```python
from build123d import *

# Parameters (mm, degrees)
EXTRUDE_1_DEPTH = 3
SKETCH_2_R      = 6.5
EXTRUDE_2_DEPTH = 0.2
SKETCH_4_W      = 3
SKETCH_4_H      = 5
EXTRUDE_3_DEPTH = 1


with BuildPart() as part:
    # 草图1 → 凸台-拉伸1 (new body)
    with BuildSketch(Plane(origin=(0, 0, 0), x_dir=(1, 0, 0), z_dir=(0, 1, 0))):
        with BuildLine():
            Line((-4.5, 7.5), (4.5, 7.5))
            ThreePointArc((4.5, 7.5), (12, 0), (4.5, -7.5))
            Line((4.5, -7.5), (-4.5, -7.5))
            ThreePointArc((-4.5, -7.5), (-12, 0), (-4.5, 7.5))
        make_face()
    extrude(amount=EXTRUDE_1_DEPTH)

    # 草图2 → 凸台-拉伸2 (add)
    with BuildSketch(Plane(origin=(0, 3, 0), x_dir=(1, 0, 0), z_dir=(0, 1, 0))):
        with Locations(Location((0, 0, 0), (0, 0, 270))):
            Circle(SKETCH_2_R)
    extrude(amount=EXTRUDE_2_DEPTH)

    # 草图4 → 凸台-拉伸3 (add)
    with BuildSketch(Plane(origin=(0, 3, 0), x_dir=(1, 0, 0), z_dir=(0, 1, 0))):
        with Locations((13.071067812, 0)):
            Rectangle(SKETCH_4_W, SKETCH_4_H)
    extrude(amount=-EXTRUDE_3_DEPTH)


solid = part.part
```
Source: CAD feature listing. Evaluate the final solid. Frame: model axes, mm. A direction names the side the tool comes from. Round coordinates to 2 decimals unless told otherwise and drop trailing zeros. Order: outer loops, then holes, each group sorted by start corner. A loop starts at its lowest first (then second) coordinate and runs counter-clockwise, first axis right, second up. Notation, with made-up numbers: (7, 31) -> (37, 31) arc R19 cw to (37, 45) -> close; hole circle Ø3 at (-6, 19.5). An arc over 180 degrees is marked (long way). One line per item, written item: value. Start each with the question number.
Q1. Section query C-C (x = 3.75). Return the cut outline in (y, z), plus the area to 3 significant figures.
Q2. Pin query (flat end, axial travel): pin 1 (1 mm diameter, centred on x = 9, y = 1.5, fed in from -Z); pin 2 (1 mm diameter, centred on x = 9, z = -4, fed in from +Y); pin 3 (0.5 mm diameter, centred on x = 13, y = 2.5, fed in from -Z). Return the tip coordinate at first contact, or that it passes through.
Q3. Section query A-A (z = 0). Return the cut outline in (x, y), plus the area to 3 significant figures.
Q4. Material intervals for probe 1 along Y at (x, z) = (2, 6.5); probe 2 along Z at (x, y) = (10.5, 0.55); probe 3 along Z at (x, y) = (8.5, 0.9), sorted ascending.
Q5. Section query D-D (z = 2.25). Return the cut outline in (x, y).
Q6. Access query for faces 1 (the flat face through (0, 1, 7.5)), 2 (the flat face through (13.1, 2.5, -2.5)), 3 (the flat face through (4.4, 3, -5.1)), 4 (the flat face through (13.1, 2.5, 2.5)). Directions: +Z, -Z, +X, -X, +Y, -Y. A direction counts if a zero-diameter tool reaches every point of the face in a straight line with its end or side. Return the directions, or none.
Q7. Section query B-B (y = 2.55). Return the cut outline in (x, z).
Findings below:
1. outline: (0, -7.5) -> (3, -7.5) -> (3, -5.31) -> (3.2, -5.31) -> (3.2, 5.31) -> (3, 5.31) -> (3, 7.5) -> (0, 7.5) -> close
1. area: 47.1 mm²
2. pin 1: z = -6.34
2. pin 2: y = 3
2. pin 3: z = -2.5
3. outline: (-12, 0) -> (12, 0) -> (12, 2) -> (14.57, 2) -> (14.57, 3) -> (6.5, 3) -> (6.5, 3.2) -> (-6.5, 3.2) -> (-6.5, 3) -> (-12, 3) -> close
3. area: 77.2 mm²
4. probe 1: 0 to 3
4. probe 2: -4.5 to 4.5
4. probe 3: -6.34 to 6.34
5. outline: (-11.65, 0) -> (11.65, 0) -> (11.65, 2) -> (14.57, 2) -> (14.57, 3) -> (6.1, 3) -> (6.1, 3.2) -> (-6.1, 3.2) -> (-6.1, 3) -> (-11.65, 3) -> close
6. face 1: +Z, +X, -X, +Y, -Y
6. face 2: -Z, +X, +Y, -Y
6. face 3: +Y
6. face 4: +Z, +X, +Y, -Y
7. outline: (-4.5, -7.5) -> (4.5, -7.5) arc R7.5 ccw to (11.57, -2.5) -> (14.57, -2.5) -> (14.57, 2.5) -> (11.57, 2.5) arc R7.5 ccw to (4.5, 7.5) -> (-4.5, 7.5) arc R7.5 ccw to start
